Part model, mm, in its own coordinate system. Face numbers are marked on the shaded views. Round coordinates to 2 decimals unless told otherwise and drop trailing zeros. Loops run counter-clockwise (first coordinate to the right, second up) from the corner with the lowest first, then second, coordinate; pieces in that order, holes last.
1) Mould opens along Z. For the marked faces 1, 2 and 3 say: +Z half, -Z half, draft (parallel to the pull), parting line (faces both ways), or undercut.
2) Band-saw the part on A-A, the plane x = 0. Write the cut outline in (y, z).
3) Probe line 1 (X direction, y = 19.5, z = 0); line 2 (Z direction, x = 2.75, y = 7.5). List the from-to ranges inside material, lowest first.
4) Drop flat-ended pins along their axis: P1, Ø1.8, axis at y = 7.5, z = 5.5, coming from the -X side; P2, Ø1.5, axis at y = 20.5, z = 1, coming from the -X side; P3, Ø0.5, axis at y = 4.5, z = -5, coming from the -X side. Give the stop position or say it passes through.
5) Band-saw the part on C-C, the plane x = -5.25. Write the cut outline in (y, z), then the cut area to 3 significant figures.
6) Band-saw the part on B-B, the plane z = 0. Write the cut outline in (x, y), then the cut area to 3 significant figures.
from build123d import *

# Parameters (mm, degrees)
ESQUISSE1_W                  = 1.5
ESQUISSE1_H                  = 30
ENL_V_MAT_EXTRU_1_DEPTH      = 7.3
ENL_V_MAT_EXTRU_1_DEPTH_BACK = 7.3


with BuildPart() as part:
    # Esquisse1 → Révolution1 (revolve)
    with BuildSketch(Plane.XY):
        with Locations((5.55, 15)):
            Rectangle(ESQUISSE1_W, ESQUISSE1_H)
    revolve(axis=Axis((0, 0, 0), (0, 1, 0)))

    # Esquisse2 → Enlèv. mat.-Extru.1 (cut, two sides)
    with BuildSketch(Plane.XY) as enl_v_mat_extru_1_sk:
        with BuildLine():
            Line((-2, -10), (-2, 10))
            ThreePointArc((-2, 10), (0, 12), (2, 10))
            Line((2, 10), (2, -10))
            ThreePointArc((2, -10), (0, -12), (-2, -10))
        make_face()
    extrude(amount=ENL_V_MAT_EXTRU_1_DEPTH, mode=Mode.SUBTRACT)
    extrude(enl_v_mat_extru_1_sk.sketch, amount=-ENL_V_MAT_EXTRU_1_DEPTH_BACK, mode=Mode.SUBTRACT)


solid = part.part
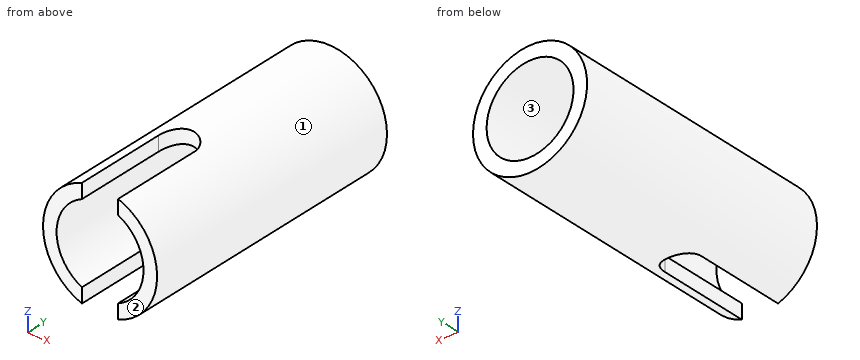
Reported:
1. face 1: parting line
1. face 2: draft
1. face 3: undercut
2. outline: (12, -6.3) - (30, -6.3) - (30, -4.8) - (12, -4.8) - close; (12, 4.8) - (30, 4.8) - (30, 6.3) - (12, 6.3) - close
3. line 1: x = -6.3 to -4.8, 4.8 to 6.3
3. line 2: z = -5.67 to -3.93, 3.93 to 5.67
4. P1: stops at x = -4.3
4. P2: stops at x = -6.3
4. P3: stops at x = -4.14
5. outline: (0, -3.48) - (30, -3.48) - (30, 3.48) - (0, 3.48) - close
5. area: 209 mm2
6. outline: (-6.3, 0) - (-4.8, 0) - (-4.8, 30) - (-6.3, 30) - close; (4.8, 0) - (6.3, 0) - (6.3, 30) - (4.8, 30) - close
6. area: 90.0 mm2
